Job drawing, mm, ordinate dimensions from the low corner. One solid piece. Coordinates: 2 decimals unless noted, no trailing zeros. Write each loop counter-clockwise with the first axis right and the second up, starting at its lowest first coordinate (ties: lowest second). Pieces come first, ordered by that corner, then holes. Notation, with made-up numbers: (57.25, 14) -> (76.25, 14) arc R8 cw to (76.25, 28) -> close; hole circle Ø7 at (70.25, 60). An arc over 180 degrees is marked (long way). One line per question, with ' | ' between items. Start each with the question number.
Item 1: Probe probe 1 along Y at (x, z) = (160.5, 3.05); probe 2 along X at (y, z) = (51.5, 5.35); probe 3 along Y at (x, z) = (194.5, 5.1). List the from-to ranges inside material, lowest first. Write a range as [from, to].
Item 2: Saw through at B-B (y = 14). List the corners of the cut face in (x, z).
Item 3: Saw through at A-A (x = 98). List the corners of the cut face in (y, z).
Item 4: Pin check, flat tips, straight feed: pin 1 (1.7 mm diameter, centred on x = 1.5, z = 1.5, fed in from -Y); pin 2 (1.7 mm diameter, centred on y = 113, z = 3.5, fed in from +X); pin 3 (3 mm diameter, centred on x = 39, z = 1.5, fed in from -Y). Stop position of each tip, or through.
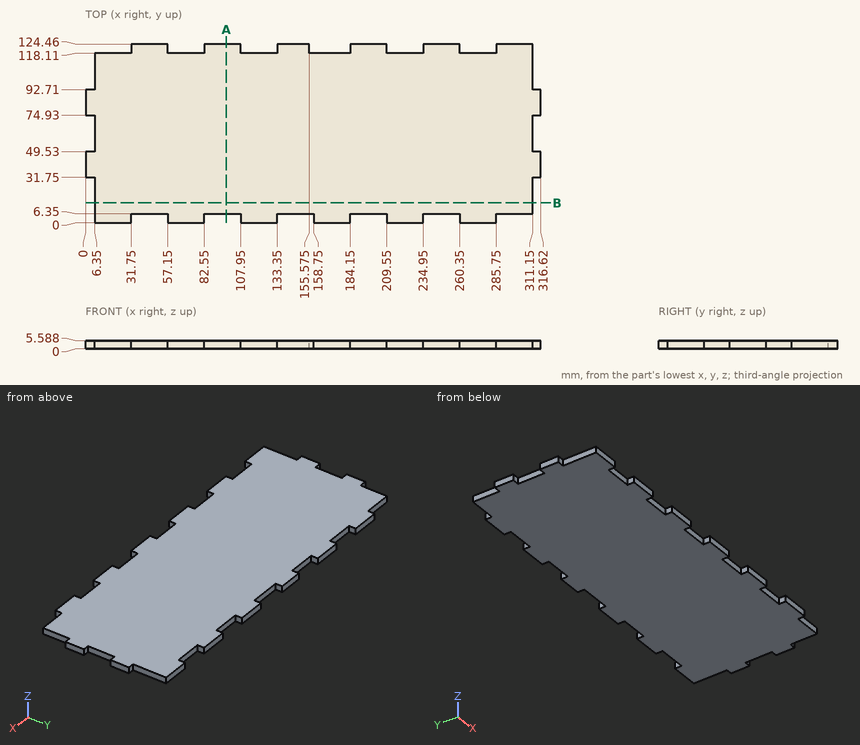
From the geometry:
1) probe 1: [0, 118.11] | probe 2: [6.35, 311.15] | probe 3: [6.35, 124.46]
2) outline: (6.35, 0) -> (311.15, 0) -> (311.15, 5.59) -> (6.35, 5.59) -> close
3) outline: (6.35, 0) -> (124.46, 0) -> (124.46, 5.59) -> (6.35, 5.59) -> close
4) pin 1: y = 31.75 | pin 2: x = 311.15 | pin 3: y = 6.35
